Job drawing, mm, ordinate dimensions from the low corner. One solid piece. Give positions to 0.01 mm unless a question says otherwise; leave off trailing zeros. Write each loop counter-clockwise with the first axis right and the second up, starting at its lowest first coordinate (ties: lowest second). Pieces come first, ordered by that corner, then holes. Notation, with made-up numbers: (70, 20) -> (102, 20) arc R16 ccw to (102, 28) -> close; hole circle Ø1 at (76, 67.25). An arc over 180 degrees is marked (long way). One line per question, with ' | ' between items. Start each with the question number.
(1) Band-saw the part on A-A, the plane y = 94. Give the cut face in (x, z) (1 decimal).
(2) Pin check, flat tips, straight feed: P1, Ø1.5, axis at x = 128, y = 71.5, coming from the -Z side (1 decimal); P2, Ø6, axis at y = 87, z = 68, coming from the +X side; P3, Ø6, axis at y = 76, z = 94.5, coming from the -X side; P4, Ø5, axis at x = 125, z = 85.5, coming from the -Y side. Stop position of each tip, or through.
(3) Band-saw the part on B-B, the plane y = 32. Give the cut face in (x, z).
(4) Drill centre lines: probe 1 along X at (y, z) = (56, 35) (1 decimal); probe 2 along Z at (x, y) = (120, 72) (1 decimal); probe 3 along Z at (x, y) = (67.5, 64). Where is each one in solid material? Low to high. Write a range as from..to.
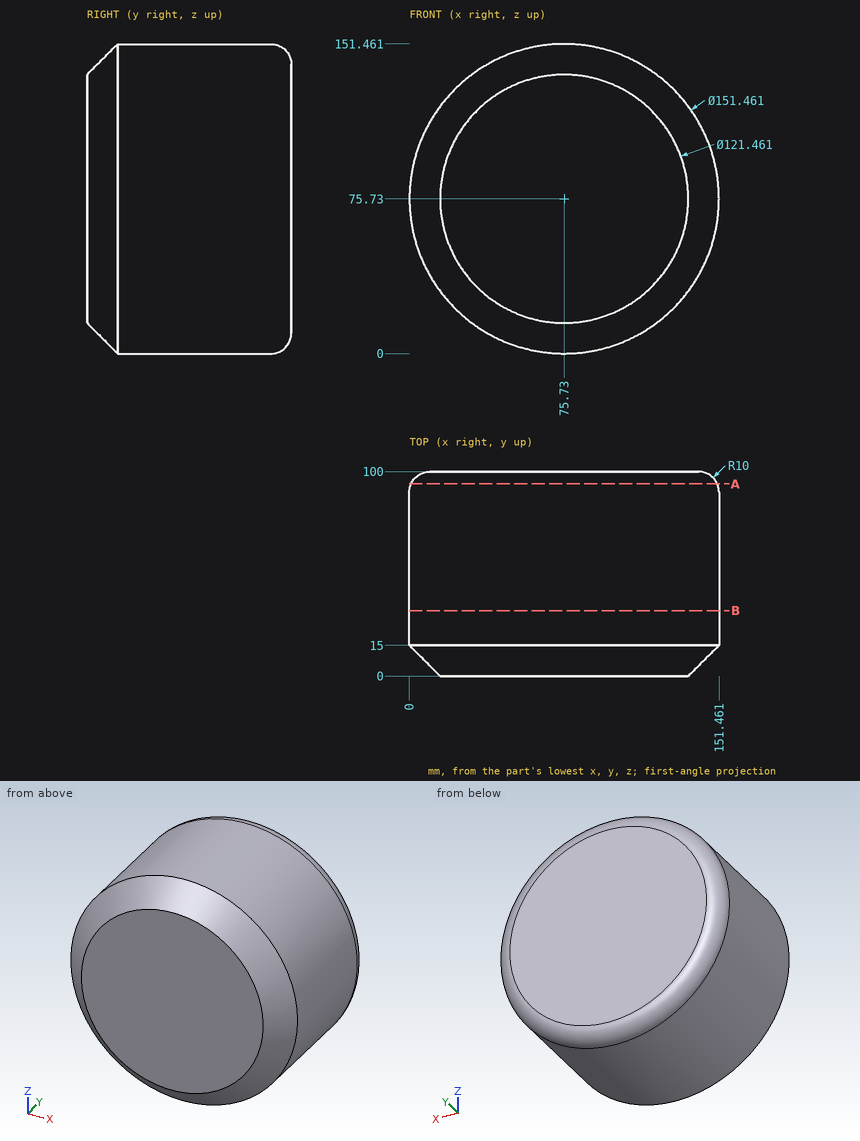
Results:
1) outline: circle Ø149.8 at (75.7, 75.7)
2) P1: stops at z = 20.2 | P2: stops at x = 151.31 | P3: stops at x = 1.66 | P4: stops at y = 0
3) outline: circle Ø151.46 at (75.73, 75.73)
4) probe 1: x = 11.9..139.6 | probe 2: z = 14.3..137.2 | probe 3: z = 0.45..151.01
